Build history of the part. All positions in model axes, mm. A direction names the side the tool comes from. Give positions to 0.01 mm unless a question says otherwise; leave off trailing zeros. Order: outer loops, then holes, each group sorted by start corner. A loop starts at its lowest first (then second) coordinate and runs counter-clockwise, first axis right, second up. Notation, with made-up numbers: (0, 33) -> (4, 33) arc R13 ccw to (4, 39) -> close; hole circle Ø10 at (-8, 5.25). An arc over 180 degrees is marked (long way). One line per item, written item: value. Start each with the question number.
(1) Saw through at B-B on x = 1.25. Give the cut face in (y, z), plus the area to 3 significant figures.
(2) Saw through at A-A on z = -35.5. Give the cut face in (x, y).
(3) Two-plate mould, pull along Y, no slides. Class faces 1 (the flat face through (2, 3, -35)), 2 (the flat face through (10, 58, -1)), 3 (the flat face through (4.6, 56.74, -65.36)): +Y half, -Y half, draft (parallel to the pull), parting line (faces both ways), or undercut.
(4) Saw through at D-D on z = -8. Give the cut face in (x, y), plus the area to 3 significant figures.
(5) Which spindle directions (+Z, -Z, +X, -X, +Y, -Y) get a long thin tool onto all of the face, cutting with end or side? Do faces 4 (the flat face through (2, 57, -40)), 5 (the flat face through (4.6, 110.36, -34.55)), 6 (the flat face through (2, 57, -67)). Say none if no direction does.
(6) Saw through at C-C on y = 27.5. Give the cut face in (x, z), plus the area to 3 significant figures.
(7) Pin check, flat tips, straight feed: pin 1 (2 mm diameter, centred on x = 3.5, y = 24, fed in from +Z); pin 2 (1.5 mm diameter, centred on x = 2, z = -34.5, fed in from +Y); pin 3 (1 mm diameter, centred on y = 23.5, z = -45.5, fed in from +X). Stop position of each tip, or through.
(8) Probe line 1 (Y direction, x = 7, z = -57); line 2 (Y direction, x = 1.1, z = -35.5); line 3 (Z direction, x = 6.75, y = 30). List the from-to ranges inside material, lowest first.
```python
from build123d import *

# Parameters (mm, degrees)
CROQUIS1_W              = 70
CROQUIS1_H              = 115
SALIENTE_EXTRUIR1_DEPTH = 10
CHAFL_N2_SIZE           = 5
VACIADO1_T              = -3
CROQUIS5_R              = 4
CROQUIS5_W              = 10
CROQUIS5_H              = 25
CORTAR_EXTRUIR1_DEPTH   = 135.810978781


with BuildPart() as part:
    # Croquis1 → Saliente-Extruir1 (new body)
    with BuildSketch(Plane(origin=(0, 0, 0), x_dir=(0, 0, -1), z_dir=(1, 0, 0))):
        with Locations((35, 57.5)):
            Rectangle(CROQUIS1_W, CROQUIS1_H)
    extrude(amount=SALIENTE_EXTRUIR1_DEPTH)

    # Chaflán2
    chafl_n2_edges = [part.edges().sort_by_distance(p)[0] for p in [
        (0, 115, -35),
        (0, 57.5, -70),
        (0, 0, -35),
        (0, 57.5, 0),
    ]]
    chamfer(chafl_n2_edges, length=CHAFL_N2_SIZE)

    # Vaciado1
    vaciado1_openings = [part.faces().sort_by_distance(p)[0] for p in [
        (10, 57.5, -35),
    ]]
    offset(amount=VACIADO1_T, openings=vaciado1_openings, kind=Kind.INTERSECTION)

    # Croquis5 → Cortar-Extruir1 (cut, through all)
    with BuildSketch(Plane(origin=(3, 0, 0), x_dir=(0, 0, -1), z_dir=(1, 0, 0))):
        with Locations((35.5, 87.5)):
            Circle(CROQUIS5_R)
        with Locations((35.5, 27.5)):
            Circle(CROQUIS5_R)
        with Locations((35, 57.5)):
            Rectangle(CROQUIS5_W, CROQUIS5_H)
    extrude(amount=-CORTAR_EXTRUIR1_DEPTH, mode=Mode.SUBTRACT)


solid = part.part
```
Results below:
1. outline: (3.75, -66.25) -> (111.25, -66.25) -> (111.25, -3.75) -> (3.75, -3.75) -> close; hole circle Ø8 at (27.5, -35.5); hole (45, -40) -> (70, -40) -> (70, -30) -> (45, -30) -> close; hole circle Ø8 at (87.5, -35.5)
1. area: 6,370 mm²
2. outline: (0, 5) -> (5, 0) -> (10, 0) -> (10, 3) -> (6.24, 3) -> (3, 6.24) -> (3, 23.5) -> (0, 23.5) -> close; (0, 31.5) -> (3, 31.5) -> (3, 45) -> (0, 45) -> close; (0, 70) -> (3, 70) -> (3, 83.5) -> (0, 83.5) -> close; (0, 91.5) -> (3, 91.5) -> (3, 108.76) -> (6.24, 112) -> (10, 112) -> (10, 115) -> (5, 115) -> (0, 110) -> close
3. face 1: -Y half
3. face 2: draft
3. face 3: undercut
4. outline: (0, 5) -> (5, 0) -> (10, 0) -> (10, 3) -> (6.24, 3) -> (3, 6.24) -> (3, 108.76) -> (6.24, 112) -> (10, 112) -> (10, 115) -> (5, 115) -> (0, 110) -> close
4. area: 373 mm²
5. face 4: +X, -X
5. face 5: +X
5. face 6: -Z, -X, +Y, -Y
6. outline: (0, -65) -> (5, -70) -> (10, -70) -> (10, -67) -> (6.24, -67) -> (3, -63.76) -> (3, -39.5) -> (0, -39.5) -> close; (0, -31.5) -> (3, -31.5) -> (3, -6.24) -> (6.24, -3) -> (10, -3) -> (10, 0) -> (5, 0) -> (0, -5) -> close
6. area: 214 mm²
7. pin 1: stops at z = -0.5
7. pin 2: stops at y = 112.75
7. pin 3: stops at x = 3
8. line 1: y = 0 to 3, 112 to 115
8. line 2: y = 3.9 to 23.5, 31.5 to 45, 70 to 83.5, 91.5 to 111.1
8. line 3: z = -70 to -67, -3 to 0
